For this review, take the finished solid that the model builds, in its own axes (mm). Round coordinates to 2 decimals unless told otherwise and drop trailing zeros. Order: outer loops, then holes, each group sorted by start corner. A loop starts at its lowest first (then second) coordinate and runs counter-clockwise, first axis right, second up. Notation, with made-up numbers: M 88,77.5 L 97,77.5 A27 ccw 97,101.5 Z; hole C 66,88 d6. An arc over 180 degrees is marked long. Answer as a JSON object with one key per item and string values.
Autodesk Fusion 360 part; units mm, degrees
sketch "草图1" plane through (0, 0, 0) normal (0, 1, 0) x (1, 0, 0)
sketch "草图2" plane through (0, 0, 0) normal (0, 1, 0) x (1, 0, 0)
  circle A0 centre (0, 0) radius 40.6099
  arc A1 (-32.8609, 18.2939) -> (-28.8479, -24.131) centre (0, 0) ccw
  arc A2 (7.2439, 36.9057) -> (-31.8644, 19.9791) centre (0, 0) ccw
  arc A3 (37.3379, 4.5151) -> (9.1546, 36.4787) centre (0, 0) ccw
  arc A4 (-27.5531, -25.5995) -> (14.0354, -34.8929) centre (0, 0) ccw
  arc A5 (15.8322, -34.1152) -> (37.5223, 2.566) centre (0, 0) ccw
  line L0 (-31.8644, 19.9791) -> (-6.1613, 14.2355)
  line L1 (-26.5994, 15.7286) -> (-7.7668, 11.5202)
  line L2 (-13.3565, -3.8268) -> (-23.1784, -20.4371)
  line L3 (-15.4427, -1.4607) -> (-28.8479, -24.131)
  line L4 (-3.3828, -15.1382) -> (14.0354, -34.8929)
  line L5 (-0.4879, -13.8853) -> (12.2743, -28.3594)
  line L6 (-26.5994, 15.7286) -> (-13.8371, 1.2545)
  line L7 (-11.7509, -1.1115) -> (-2.5741, -11.5193)
  line L8 (-32.8609, 18.2939) -> (-15.4427, -1.4607)
  line L9 (-13.3565, -3.8268) -> (-5.469, -12.7722)
  line L10 (-3.3828, -15.1382) -> (-27.5531, -25.5995)
  line L11 (-5.469, -12.7722) -> (-23.1784, -20.4371)
  line L12 (10.4571, -9.1481) -> (12.2743, -28.3594)
  line L13 (13.352, -7.8952) -> (15.8322, -34.1152)
  line L14 (30.7644, 2.91) -> (13.0549, -4.7548)
  line L15 (10.1601, -6.0078) -> (-2.5741, -11.5193)
  line L16 (37.5223, 2.566) -> (13.352, -7.8952)
  line L17 (10.4571, -9.1481) -> (-0.4879, -13.8853)
  line L18 (-4.6884, 10.8323) -> (8.8534, 7.8063)
  line L19 (11.9318, 7.1184) -> (30.7644, 2.91)
  line L20 (-3.0828, 13.5475) -> (8.5563, 10.9467)
  line L21 (11.6348, 10.2587) -> (37.3379, 4.5151)
  line L22 (6.7391, 30.1579) -> (8.5563, 10.9467)
  line L23 (8.8534, 7.8063) -> (10.1601, -6.0078)
  line L24 (9.1546, 36.4787) -> (11.6348, 10.2587)
  line L25 (11.9318, 7.1184) -> (13.0549, -4.7548)
  line L26 (6.7391, 30.1579) -> (-3.0828, 13.5475)
  line L27 (-4.6884, 10.8323) -> (-11.7509, -1.1115)
  line L28 (7.2439, 36.9057) -> (-6.1613, 14.2355)
  line L29 (-7.7668, 11.5202) -> (-13.8371, 1.2545)
extrude "拉伸1" add sketch "草图2" along normal blind 5 makes body 1
sketch "草图3" plane through (0, 0, 0) normal (0, 1, 0) x (1, 0, 0)
  circle A0 centre (-95, 0) radius 2.5
  circle A1 centre (-95, 0) radius 4
  dimension "d6" = 5
  dimension "d7" = 8
extrude "拉伸2" add sketch "草图3" along normal blind 5 separate body makes body 2
move_body "移动1" bodies 2 to x (1, 0, 0) y (0, 1, 0) z (0, 0, 1) at (54.5157, 0, 0.7678)
move_body "移动2" bodies 2 to x (1, 0, 0) y (0, 1, 0) z (0, 0, 1) at (-1.1104, 0, 0.0218)
combine "合并1" operation add target body 1 tool bodies 2
1) Add section B-B on z = 17. State the section outline as (x, y) points.
Geometry check:
{"outline": "M -36.88,0 L -33.55,0 L -33.55,5 L -36.88,5 Z; M -24.63,0 L -21.15,0 L -21.15,5 L -24.63,5 Z; M -15.24,0 L -7.68,0 L -7.68,5 L -15.24,5 Z; M -1.74,0 L 2.26,0 L 2.26,5 L -1.74,5 Z; M 11.2,0 L 14.21,0 L 14.21,5 L 11.2,5 Z; M 33.55,0 L 36.88,0 L 36.88,5 L 33.55,5 Z"}
2) Insertion check: P1, Ø1.5, axis at x = -11, y = 0.5, coming from the +Z side; P2, Ø2, axis at x = 15, z = -12, coming from the +Y side; P3, Ø1.5, axis at y = 2.5, z = -4, coming from the -X side. Each pin has a flat end and moves straight along its axis. Give the tip position at first contact, or say it passes through.
Geometry check:
{"P1": "stops at z = 39.3", "P2": "passes through", "P3": "stops at x = -40.48"}
3) Add section A-A on x = 20.5. State the section outline as (y, z) points, and give its area (3 significant figures).
Geometry check:
{"outline": "M 0,-35.06 L 5,-35.06 L 5,-31.53 L 0,-31.53 Z; M 0,-8.28 L 5,-8.28 L 5,-5.2 L 0,-5.2 Z; M 0,1.53 L 5,1.53 L 5,4.8 L 0,4.8 Z; M 0,31.53 L 5,31.53 L 5,35.06 L 0,35.06 Z", "area": "67.0 mm²"}
4) Add section D-D on z = -32. State the section outline as (x, y) points, and give its area (3 significant figures).
Geometry check:
{"outline": "M -25,0 L -19.76,0 L -19.76,5 L -25,5 Z; M 4.34,0 L 9.58,0 L 9.58,5 L 4.34,5 Z; M 19.76,0 L 25,0 L 25,5 L 19.76,5 Z", "area": "78.6 mm²"}
5) Add section C-C on x = -22. State the section outline as (y, z) points, and give its area (3 significant figures).
Geometry check:
{"outline": "M 0,-34.13 L 5,-34.13 L 5,-30.5 L 0,-30.5 Z; M 0,-17.77 L 5,-17.77 L 5,-14.7 L 0,-14.7 Z; M 0,-10.51 L 5,-10.51 L 5,-5.98 L 0,-5.98 Z; M 0,12.55 L 5,12.55 L 5,18.44 L 0,18.44 Z; M 0,19.93 L 5,19.93 L 5,23.2 L 0,23.2 Z; M 0,30.5 L 5,30.5 L 5,34.13 L 0,34.13 Z", "area": "120 mm²"}
6) Mouldability with a two-part tool opening along X and no side actions: class faces 1 (the flat face through (-22.051, 2.465, 12.637)), 2 (the flat face through (4, 5, 9)), 3 (the cylindrical face through (-44.09, 2.46, 0.91)) as +X half, -X half, draft (parallel to the pull), parting line (faces both ways), or undercut.
Geometry check:
{"face 1": "undercut", "face 2": "draft", "face 3": "undercut"}
7) For L1, parallel to Z at x = -8.5, y = 1.7; L2, parallel to X at y = 2.95, z = 14.5; L3, parallel to X at y = 4.8, z = 18.5, list the stretches that pass through material, from the lowest coordinate up.
Geometry check:
{"L1": "z = -39.71 to -36.64, -14.76 to -11.68, -10.28 to -4.39, 4.8 to 9.33, 14.08 to 17.35, 36.64 to 39.71", "L2": "x = -37.93 to -34.7, -23.15 to -19.67, -9.46 to 0.05, 10.96 to 13.98, 34.7 to 37.93", "L3": "x = -36.15 to -32.75, -25.52 to -22.03, -18.7 to -11.15, -0.42 to 3.58, 11.34 to 14.36, 32.75 to 36.15"}
